from build123d import *

# Parameters (mm, degrees)
F0_W     = 45
F0_H     = 1407
F1_DEPTH = 22.5
F3_SIZE2 = 44.99999
F3_SIZE  = 44.99999
F2_W     = 16.4
F2_H     = 45
F4_DEPTH = 45
F5_R     = 9
F6_DEPTH = 45.001
F7_DEPTH = 15
F9_D     = 3.5
F9_DEPTH = 30
F9_TIP   = 1.0515060833


# Not quite as in the source:
# - a fillet or chamfer is up to 0.001 mm smaller than in the source, because OpenCascade refuses the exact size


with BuildPart() as f1:
    # F0 (on Front) → F1 (new body, symmetric)
    with BuildSketch(Plane.XZ):
        with Locations((0, -490.1653682211)):
            Rectangle(F0_W, F0_H)
    extrude(amount=F1_DEPTH, both=True)

    # F3 (size 45 and 45 in the source; OpenCascade refuses exactly that, so slightly less here)
    f3_edges = [f1.edges().sort_by_distance(p)[0] for p in [
        (0, 22.5, 213.334632),
    ]]
    chamfer(f3_edges, length=F3_SIZE, length2=F3_SIZE2)

    # F2 (on face) → F4 (cut)
    with BuildSketch(Plane.XY.offset(213.3346317789)):
        Rectangle(F2_W, F2_H)
    extrude(amount=-F4_DEPTH, mode=Mode.SUBTRACT)

    # F5 (on face) → F6 (cut, through all)
    with BuildSketch(Plane(origin=(-22.5, 0, 0), x_dir=(0, -1, 0), z_dir=(-1, 0, 0))):
        with Locations((0, 38.3346317789)):
            Circle(F5_R)
        with Locations((0, -311.6653682211)):
            Circle(F5_R)
        with Locations((0, -661.6653682211)):
            Circle(F5_R)
        with Locations((0, -1011.6653682211)):
            Circle(F5_R)
    extrude(amount=-F6_DEPTH, mode=Mode.SUBTRACT)

    # F5 (on face) → F7 (join)
    with BuildSketch(Plane(origin=(-22.5, 0, 0), x_dir=(0, -1, 0), z_dir=(-1, 0, 0))):
        with Locations((0, -1011.6653682211)):
            Circle(F5_R)
        with Locations((0, -661.6653682211)):
            Circle(F5_R)
        with Locations((0, -311.6653682211)):
            Circle(F5_R)
        with Locations((0, 38.3346317789)):
            Circle(F5_R)
    extrude(amount=-F7_DEPTH)

    # F9
    with Locations(Plane(origin=(0, 22.5, 0), x_dir=(-1, 0, 0), z_dir=(0, 1, 0))):
        with Locations((10, 143.3346317789), (10, 103.3346317789), (10, 63.3346317789), (-10, 63.3346317789), (-10, 103.3346317789), (-10, 143.3346317789)):
            Hole(F9_D / 2, depth=F9_DEPTH)
            with Locations((0, 0, -(F9_DEPTH + F9_TIP / 2))):  # 118° drill point
                Cone(0, F9_D / 2, F9_TIP, mode=Mode.SUBTRACT)


solid = f1.part
Verification items for the finished model (mm, model axes). Give positions to 0.01 mm unless a question says otherwise; leave off trailing zeros. Answer as CSV lines item,"result".
Q1. Sectioned sample at A-A on y = 0. Count the separate pieces of the cut face and the enclosed holes in it, plus the area to 3 significant figures.
Solutions:
separate pieces,"1"
enclosed holes,"6"
area,"59,700 mm²"
Q2. Scan lines: probe 1 along Y at (x, z) = (1, 38.5); probe 2 along Z at (x, y) = (12, 0); probe 3 along Z at (x, y) = (7, 7). Record each from-to range of solid material in increasing order.
Solutions:
probe 1,"y = -22.5 to -9, 9 to 22.5"
probe 2,"z = -1193.67 to -1020.67, -1002.67 to -670.67, -652.67 to -320.67, -302.67 to 29.33, 47.33 to 190.83"
probe 3,"z = -1193.67 to -1017.32, -1006.01 to -667.32, -656.01 to -317.32, -306.01 to 32.68, 43.99 to 168.33"
Q3. Depth check by flat-ended pin: pin 1 (5 mm diameter, centred on x = -17, y = -5.5, fed in from +Z); pin 2 (1.5 mm diameter, centred on x = 10.5, y = -18, fed in from +Z); pin 3 (4 mm diameter, centred on x = 10, z = 143.33, fed in from +Y); pin 4 (5.5 mm diameter, centred on y = -2.5, z = -1010, fed in from +X). Enter the tip coordinate at first touch or a pass-through.
Solutions:
pin 1,"stops at z = 198.83"
pin 2,"stops at z = 209.58"
pin 3,"stops at y = 22.5"
pin 4,"stops at x = -7.5"
Q4. Release check for a two-part mould opening along X. For faces 1 (the flat face through (0, -22.5, -480)), 2 (the flat face through (-8.2, -5, 186)), 3 (the flat face through (-22.5, 0, -480)), 4 (the flat face through (8.2, -5, 186)) record: +X half, -X half, draft (parallel to the pull), parting line (faces both ways), or undercut.
Solutions:
face 1,"draft"
face 2,"undercut"
face 3,"-X half"
face 4,"undercut"
